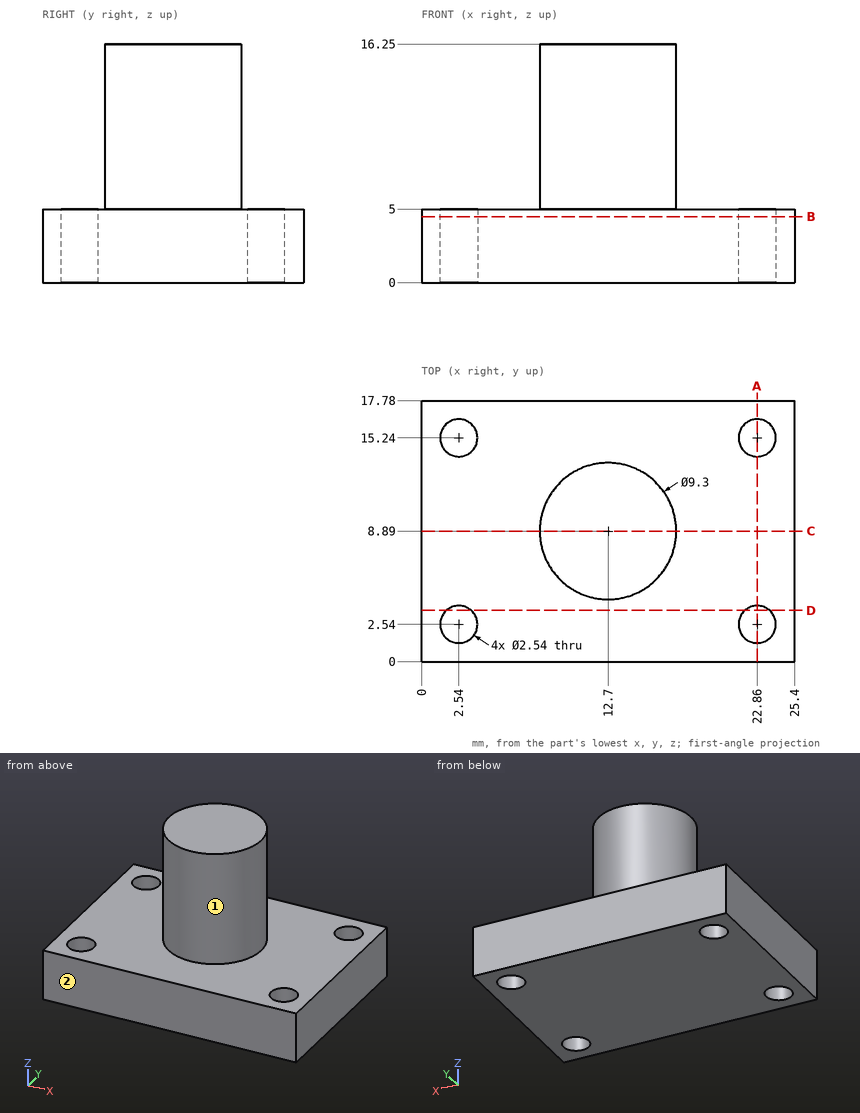
Can you work these out from the drawing? Everything is in mm from the part's minimum corner. A direction names the side the tool comes from. Round coordinates to 2 decimals unless told otherwise and drop trailing zeros. Loops run counter-clockwise (first coordinate to the right, second up) from the corner with the lowest first, then second, coordinate; pieces in that order, holes last. Notation, with made-up numbers: (20, -26.75) - (59, -26.75) arc R12 cw to (59, -13.75) - close; hole circle Ø4 at (-16.75, 85.25). An arc over 180 degrees is marked (long way). Answer in a Markdown table with one row per item. Add a question column.
(1) I need wall thicknesses on line 1 along Y through (x, z) = (2.54, 1.4); line 2 along Z through (x, y) = (19.75, 6.75); line 3 along Y through (x, z) = (15.5, 8.75). Which ranges of each line are inside material? Lowest first, please.
(2) If we section it at A-A (x = 22.86): Please give me the cut outline in (y, z), plus the area to 3 significant figures.
(3) For the marked faces 1 and 2, which set-ups out of +Z, -Z, +X, -X, +Y, -Y let a thin tool reach every point of the face, with its end or its side?
(4) If we section it at C-C (y = 8.89): Please give me the cut outline in (x, z).
(5) If we section it at D-D (y = 3.5): Please give me the cut outline in (x, z).
(6) I'm going to push flat-ended pins straight in: pin 1 (1.5 mm diameter, centred on x = 7, y = 12.5, fed in from -Z); pin 2 (3 mm diameter, centred on y = 11, z = 10.5, fed in from +X). Where does each tip first touch, or does it pass through?
(7) If we section it at B-B (z = 4.5): Please give me the cut outline in (x, y), plus the area to 3 significant figures.
Model answer:
| question | item | result |
|---|---|---|
| 1 | line 1 | y = 0 to 1.27, 3.81 to 13.97, 16.51 to 17.78 |
| 1 | line 2 | z = 0 to 5 |
| 1 | line 3 | y = 5.18 to 12.6 |
| 2 | outline | (0, 0) - (1.27, 0) - (1.27, 5) - (0, 5) - close; (3.81, 0) - (13.97, 0) - (13.97, 5) - (3.81, 5) - close; (16.51, 0) - (17.78, 0) - (17.78, 5) - (16.51, 5) - close |
| 2 | area | 63.5 mm² |
| 3 | face 1 | +Z |
| 3 | face 2 | +Z, -Z, +X, -X, -Y |
| 4 | outline | (0, 0) - (25.4, 0) - (25.4, 5) - (17.35, 5) - (17.35, 16.25) - (8.05, 16.25) - (8.05, 5) - (0, 5) - close |
| 5 | outline | (0, 0) - (1.71, 0) - (1.71, 5) - (0, 5) - close; (3.37, 0) - (22.03, 0) - (22.03, 5) - (3.37, 5) - close; (23.69, 0) - (25.4, 0) - (25.4, 5) - (23.69, 5) - close |
| 6 | pin 1 | stops at z = 0 |
| 6 | pin 2 | stops at x = 17.31 |
| 7 | outline | (0, 0) - (25.4, 0) - (25.4, 17.78) - (0, 17.78) - close; hole circle Ø2.54 at (2.54, 2.54); hole circle Ø2.54 at (2.54, 15.24); hole circle Ø2.54 at (22.86, 2.54); hole circle Ø2.54 at (22.86, 15.24) |
| 7 | area | 431 mm² |
